Job drawing, mm, ordinate dimensions from the low corner. One solid piece. Round coordinates to 2 decimals unless told otherwise and drop trailing zeros. Write each loop counter-clockwise with the first axis right and the second up, starting at its lowest first coordinate (ties: lowest second). Pieces come first, ordered by that corner, then holes.
1) Wall check: probe 1 along Y at (x, z) = (30, 3); probe 2 along Y at (x, z) = (36, 1.55); probe 3 along X at (y, z) = (176, 4.75). Give the ranges that are in metal, low to high.
2) Saw through at C-C (z = 1.45). Write the cut outline in (x, y), plus the area to 3 significant figures.
3) Saw through at A-A (y = 180). Write the cut outline in (x, z), plus the area to 3 significant figures.
4) Saw through at B-B (x = 30). Write the cut outline in (y, z).
5) Flat gauge pin, fed straight in: pin 1 (8.5 mm diameter, centred on x = 30, y = 180, fed in from +Z). Where does the tip first touch, or does it go through?
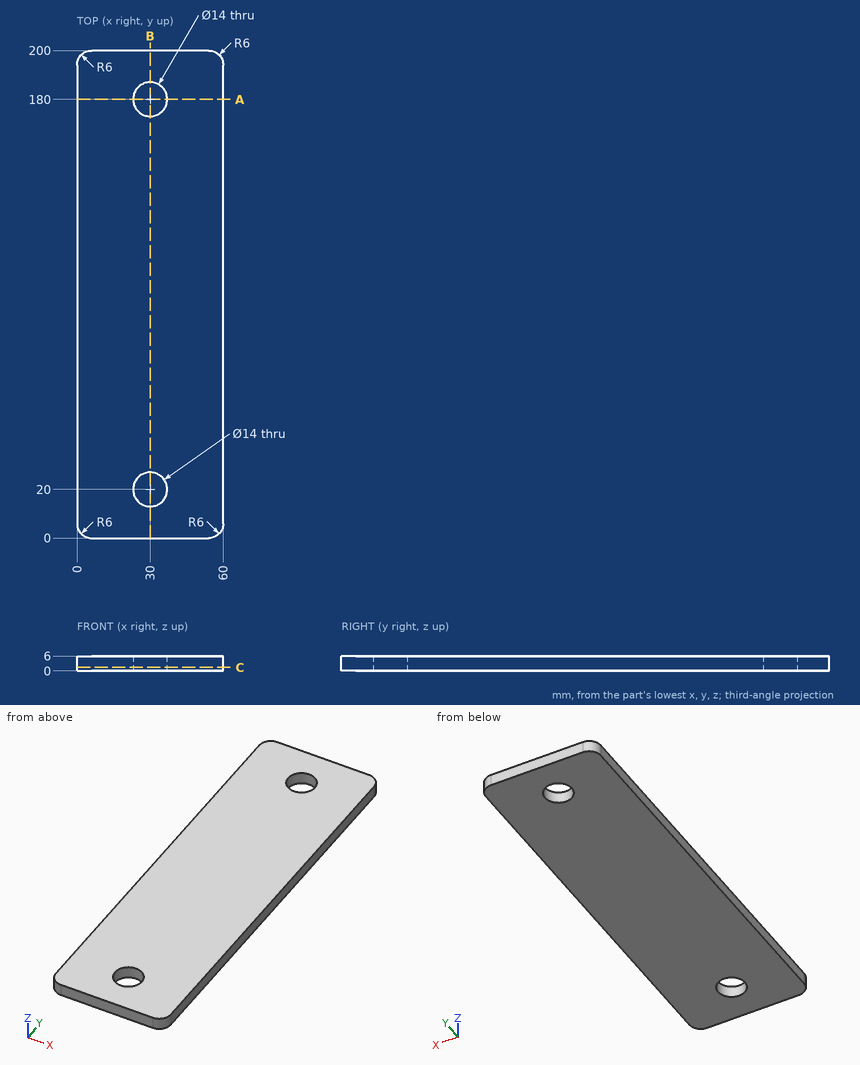
Evaluation:
1. probe 1: y = 0 to 13, 27 to 173, 187 to 200
1. probe 2: y = 0 to 16.39, 23.61 to 176.39, 183.61 to 200
1. probe 3: x = 0 to 24.26, 35.74 to 60
2. outline: (0, 6) arc R6 ccw to (6, 0) - (54, 0) arc R6 ccw to (60, 6) - (60, 194) arc R6 ccw to (54, 200) - (6, 200) arc R6 ccw to (0, 194) - close; hole circle Ø14 at (30, 20); hole circle Ø14 at (30, 180)
2. area: 11,700 mm2
3. outline: (0, 0) - (23, 0) - (23, 6) - (0, 6) - close; (37, 0) - (60, 0) - (60, 6) - (37, 6) - close
3. area: 276 mm2
4. outline: (0, 0) - (13, 0) - (13, 6) - (0, 6) - close; (27, 0) - (173, 0) - (173, 6) - (27, 6) - close; (187, 0) - (200, 0) - (200, 6) - (187, 6) - close
5. pin 1: passes through
